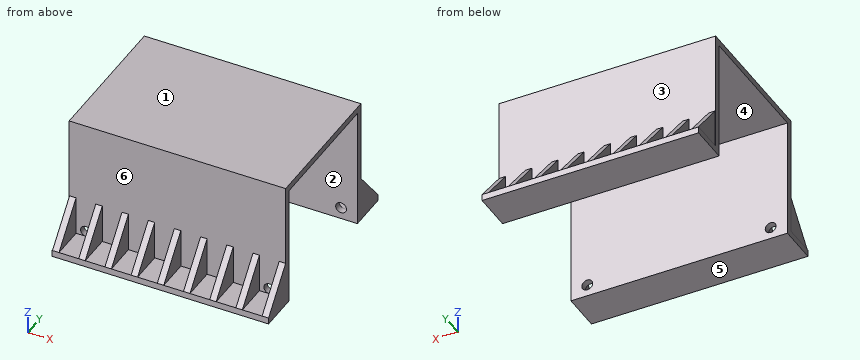
from build123d import *

# Parameters (mm, degrees)
SKETCH1_W                = 100
SKETCH1_H                = 60
BOSS_EXTRUDE1_DEPTH      = 3
SKETCH2_W                = 100
SKETCH2_H                = 3
BOSS_EXTRUDE2_DEPTH      = 53
BOSS_EXTRUDE2_DEPTH_BACK = 3
SKETCH3_W                = 100
SKETCH3_H                = 18
BOSS_EXTRUDE3_DEPTH      = 3
BOSS_EXTRUDE4_DEPTH      = 3
SKETCH6_W                = 97
SKETCH6_H                = 18
BOSS_EXTRUDE5_DEPTH      = 3
LPATTERN4_COUNT          = 9
LPATTERN4_PITCH          = 12.1
SKETCH7_R                = 2.5
CUT_EXTRUDE2_DEPTH       = 82
CUT_EXTRUDE4_DEPTH       = 101


with BuildPart() as part:
    # Sketch1 → Boss-Extrude1 (new body)
    with BuildSketch(Plane.XY):
        with Locations((50, 30)):
            Rectangle(SKETCH1_W, SKETCH1_H)
    extrude(amount=BOSS_EXTRUDE1_DEPTH)

    # Sketch2 → Boss-Extrude2 (add, two sides)
    with BuildSketch(Plane(origin=(0, 0, 0), x_dir=(-1, 0, 0), z_dir=(0, 0, -1))) as boss_extrude2_sk:
        with Locations((-50, 61.5)):
            Rectangle(SKETCH2_W, SKETCH2_H)
        with Locations((-50, -1.5)):
            Rectangle(SKETCH2_W, SKETCH2_H)
    extrude(amount=BOSS_EXTRUDE2_DEPTH)
    extrude(boss_extrude2_sk.sketch, amount=-BOSS_EXTRUDE2_DEPTH_BACK)

    # Sketch3 → Boss-Extrude3 (add)
    with BuildSketch(Plane(origin=(0, 0, -53), x_dir=(-1, 0, 0), z_dir=(0, 0, -1))):
        with Locations((-50, 69)):
            Rectangle(SKETCH3_W, SKETCH3_H)
        with Locations((-50, -9)):
            Rectangle(SKETCH3_W, SKETCH3_H)
    extrude(amount=BOSS_EXTRUDE3_DEPTH)

    # Sketch5 → Boss-Extrude4 (add)
    with BuildSketch(Plane(origin=(100, 0, 0), x_dir=(0, 0, -1), z_dir=(1, 0, 0))):
        Polygon((35, -3), (53, -3), (53, -18), align=None)
    boss_extrude4 = extrude(amount=-BOSS_EXTRUDE4_DEPTH)

    # Sketch6 → Boss-Extrude5 (add)
    with BuildSketch(Plane.XZ.offset(3)):
        with Locations((48.5, -44)):
            Rectangle(SKETCH6_W, SKETCH6_H)
    extrude(amount=-BOSS_EXTRUDE5_DEPTH)

    # LPattern4: Boss-Extrude4 ×9
    with Locations(*[(-i * LPATTERN4_PITCH, 0, 0) for i in range(1, LPATTERN4_COUNT)]):
        add(boss_extrude4)

    # Sketch7 → Cut-Extrude2 (cut, through all)
    with BuildSketch(Plane.XZ.offset(3)):
        with Locations((92.45, -50.5)):
            Circle(SKETCH7_R)
        with Locations((7.75, -50.5)):
            Circle(SKETCH7_R)
    extrude(amount=-CUT_EXTRUDE2_DEPTH, mode=Mode.SUBTRACT)

    # Sketch10 → Cut-Extrude4 (cut, through all)
    with BuildSketch(Plane.ZY):
        Polygon((0, 30), (3, 30), (3, 114.137691369), (-76.856579816, 109.737899985), (-70.799886201, 33.223019627), align=None)
    extrude(amount=-CUT_EXTRUDE4_DEPTH, mode=Mode.SUBTRACT)

    # Mirror2: part across plane


with BuildPart() as part_1:
    add(part.part)
    add(part.part.mirror(Plane(origin=(100, 30, 0), x_dir=(0, 0, 1), z_dir=(0, -1, 0))))


solid = part_1.part
Geometry check sheet. Reference: the model listing, model coordinates, mm. Face numbers are marked on the shaded views. A direction names the side the tool comes from. Round coordinates to 2 decimals unless told otherwise and drop trailing zeros. Order: outer loops, then holes, each group sorted by start corner. A loop starts at its lowest first (then second) coordinate and runs counter-clockwise, first axis right, second up. Notation, with made-up numbers: (35.25, -12.5) - (79.25, -12.5) arc R11 ccw to (79.25, -7.5) - close; hole circle Ø2 at (10.25, 79.5). An arc over 180 degrees is marked (long way). One line per question, with ' | ' between items. Start each with the question number.
(1) Sectioned sample at C-C on y = 31. Record the cut outline in (x, z).
(2) Sectioned sample at A-A on z = -16.5. Record the cut outline in (x, y), and give its area (3 significant figures).
(3) Depth check by flat-ended pin: pin 1 Ø4 at (x, z) = (40, -32.5) entering from -Y; pin 2 Ø4.5 at (x, y) = (80.5, -7) entering from +Z; pin 3 Ø2 at (x, z) = (27.5, -24) entering from +Y. Enter the tip coordinate at first touch or a pass-through.
(4) Thickness scan on L1, parallel to X at y = -0.8, z = -50.5; L2, parallel to Y at x = 21.5, z = -26; L3, parallel to Z at x = 92.45, y = -1.6. Record the ranges inside material, lowest first. Write a range as [from, to].
(5) Sectioned sample at D-D on z = -50.5. Count the separate pieces of the cut face and the enclosed holes in it, and give its area (3 significant figures).
(6) Release check for a two-part mould opening along Y. For the marked faces 1, 2 and 3 record: released by +Y, released by -Y, zero draft, split by the parting line, or undercut.
(7) Sectioned sample at B-B on x = 44. Record the cut outline in (y, z), and give its area (3 significant figures).
(8) Access from +Z, -Z, +X, -X, +Y, -Y to the whole of each face (thin tool, end or side, straight path). Record for the marked faces 4, 5 and 6.
Conclusion:
1) outline: (0, 0) - (100, 0) - (100, 3) - (0, 3) - close
2) outline: (0, -3) - (100, -3) - (100, 0) - (0, 0) - close; (0, 60) - (100, 60) - (100, 63) - (0, 63) - close | area: 600 mm2
3) pin 1: stops at y = -3 | pin 2: stops at z = -53 | pin 3: stops at y = 63
4) L1: x = [0, 5.25], [10.25, 89.95], [94.95, 100] | L2: y = [-3, 0], [60, 63] | L3: z = [-56, -53], [-48, 3]
5) separate pieces: 6 | enclosed holes: 0 | area: 1,240 mm2
6) face 1: zero draft | face 2: undercut | face 3: released by +Y
7) outline: (-18, -56) - (0, -56) - (0, 0) - (60, 0) - (60, -56) - (78, -56) - (78, -53) - (63, -53) - (63, 3) - (-3, 3) - (-3, -53) - (-18, -53) - close | area: 624 mm2
8) face 4: -Z, +X, -X | face 5: -Z, +X, -X, +Y, -Y | face 6: +Z, -Y
